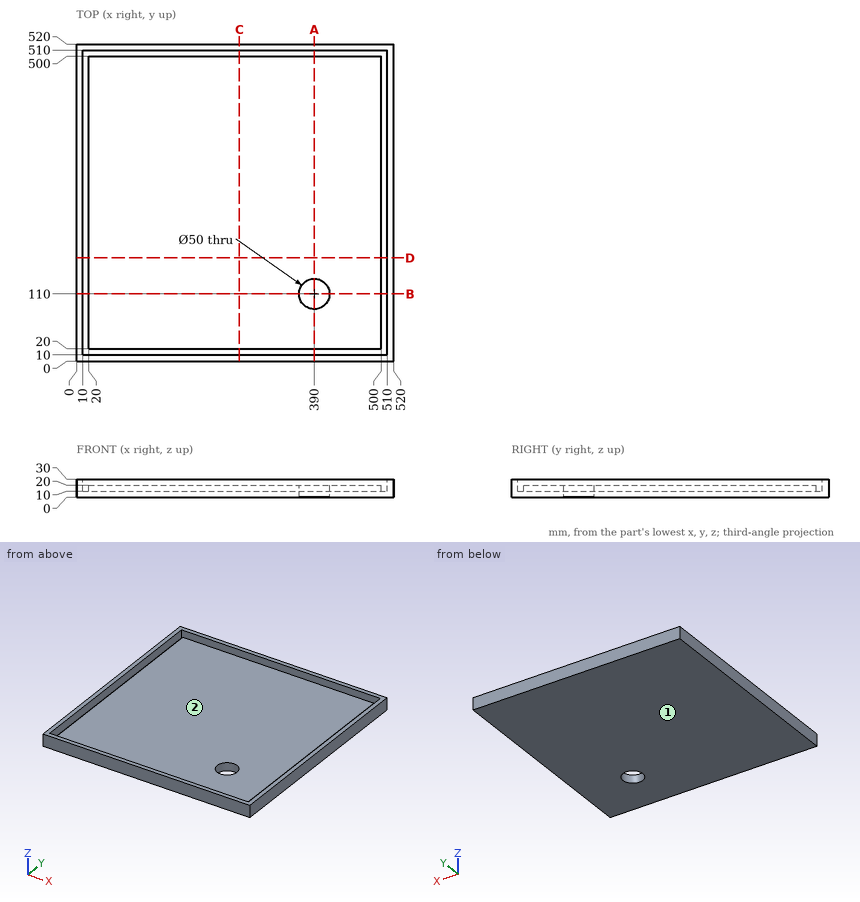
Check sheet for the drawn part. Datum: minimum x, y, z corner. Units: mm. Give positions to 0.01 mm unless a question says otherwise; leave off trailing zeros. Write each loop counter-clockwise with the first axis right and the second up, starting at its lowest first coordinate (ties: lowest second). Pieces come first, ordered by that corner, then holes. Notation, with made-up numbers: M -38,48 L -20,48 A15 ccw -20,71 Z; hole C 37.25,-1.5 d7. An arc over 180 degrees is marked long. Write item = value, one per line.
(1) Material ranges on line 1 (X direction, y = 489, z = 16); line 2 (Y direction, x = 390, z = 16); line 3 (Y direction, x = 390, z = 8.25), recorded low to high.
Found:
line_1 = 0 to 10, 20 to 500, 510 to 520
line_2 = 0 to 10, 20 to 85, 135 to 500, 510 to 520
line_3 = 0 to 85, 135 to 520
(2) Sectioned sample at C-C (x = 267). Record the cut outline in (y, z).
Found:
outline = M 0,0 L 520,0 L 520,30 L 510,30 L 510,10 L 500,10 L 500,20 L 20,20 L 20,10 L 10,10 L 10,30 L 0,30 Z
(3) Sectioned sample at B-B (y = 110). Record the cut outline in (x, z).
Found:
outline = M 0,0 L 365,0 L 365,20 L 20,20 L 20,10 L 10,10 L 10,30 L 0,30 Z; M 415,0 L 520,0 L 520,30 L 510,30 L 510,10 L 500,10 L 500,20 L 415,20 Z
(4) Draft check along Y on the marked faces 1 and 2. Enter one of: released by +Y, released by -Y, zero draft, split by the parting line, or undercut.
Found:
face_1 = zero draft
face_2 = undercut
(5) Sectioned sample at A-A (x = 390). Record the cut outline in (y, z), then the cut area to 3 significant figures.
Found:
outline = M 0,0 L 85,0 L 85,20 L 20,20 L 20,10 L 10,10 L 10,30 L 0,30 Z; M 135,0 L 520,0 L 520,30 L 510,30 L 510,10 L 500,10 L 500,20 L 135,20 Z
area = 9,400 mm2
(6) Go/stop test with a flat-tipped pin: pin 1 Ø8 at (x, y) = (467.5, 383.5) entering from +Z. Record where the tip stops, or that it passes through.
Found:
pin_1 = 20
